Verification items for the finished model (mm, model axes). A direction names the side the tool comes from. Coordinates: 2 decimals unless noted, no trailing zeros. Loops run counter-clockwise (first coordinate to the right, second up) from the corner with the lowest first, then second, coordinate; pieces in that order, holes last. Notation, with made-up numbers: (6, 81) -> (44, 81) arc R17 cw to (44, 101) -> close; hole circle Ø10 at (20.25, -1.75). An arc over 180 degrees is marked (long way). Answer as a JSON object with one key per item and string values. Group by question number.
Q1. Set-up check for faces 1 (the flat face through (-2.938, 0, 37)), 2 (the flat face through (-1, 0, 65)), 3 (the flat face through (2.938, 0, 26)): record each of +Z, -Z, +X, -X, +Y, -Y from which the full face is reachable in a straight line by a thin tool's end or side.
Q2. Gauge pin test, flat ends, axial feed: pin 1 Ø2 at (x, y) = (6, 0.5) entering from +Z; pin 2 Ø2.5 at (x, z) = (-7, 0.83) entering from -Y; pin 3 Ø2.5 at (y, z) = (0, 20.5) entering from +X. Record the tip position at first contact, or that the pin passes through.
Q3. Cross-section at A-A on x = -7. Record the boundary of the cut face in (y, z).
Q4. Cross-section at C-C on y = -1.1. Give the number of separate pieces and of enclosed holes in the cut face, and give its area (3 significant figures).
Q5. Scan lines: L1, parallel to X at y = -0.1, z = 11; L2, parallel to Z at x = -7, y = 2; L3, parallel to Z at x = -0.5, y = 2.1. Record each from-to range of solid material in increasing order.
Q6. Release check for a two-part mould opening along X. For faces 4 (the cylindrical face through (-0.115, -0.035, -0.424)), 5 (the cylindrical face through (4.82, -0.04, 5.92)), 6 (the flat face through (1, -2.5, 26)) record: released by +X, released by -X, zero draft, split by the parting line, or undercut.
Q7. Cross-section at D-D on x = -1.25. Record the boundary of the cut face in (y, z).
Q8. Cross-section at B-B on z = 19. Record the boundary of the cut face in (x, y).
```python
from build123d import *

# Parameters (mm, degrees)
BOSS_EXTRU_1_DEPTH      = 2.5
BOSS_EXTRU_1_DEPTH_BACK = 2.5
ESQUISSE1_R             = 1.5


with BuildPart() as part:
    # Esquisse1 → Boss.-Extru.1 (new, two sides: drawn at the far end of the back side and taken through both)
    with BuildSketch(Plane(origin=(0, 0, 0), x_dir=(1, 0, 0), z_dir=(0, 1, 0)).offset(-BOSS_EXTRU_1_DEPTH_BACK)):
        with BuildLine():
            Line((1.688009203, -65), (-2.938009191, -65))
            Line((-2.938009191, -65), (-2.938009191, -9.008494736))
            ThreePointArc((-2.938009191, -9.008494736), (-4.78031572, -5.95992834), (-7.884337553, -4.212673672))
            ThreePointArc((-7.884337553, -4.212673672), (-10.499981587, -0.814885018), (-7.862349987, 2.565863566))
            ThreePointArc((-7.862349987, 2.565863566), (0, 0.423762079), (7.862349987, 2.565863566))
            ThreePointArc((7.862349987, 2.565863566), (10.499981587, -0.814885018), (7.884337553, -4.212673672))
            ThreePointArc((7.884337553, -4.212673672), (4.78031572, -5.95992834), (2.938009191, -9.008494736))
            Line((2.938009191, -9.008494736), (2.938009191, -43.679635922))
            ThreePointArc((2.938009191, -43.679635922), (2.839937622, -43.977047315), (2.584195047, -44.1577883))
            Line((2.584195047, -44.1577883), (2.041823351, -44.323607971))
            ThreePointArc((2.041823351, -44.323607971), (1.688009203, -44.801760349), (2.041823351, -45.279912727))
            Line((2.041823351, -45.279912727), (2.584195044, -45.445732395))
            ThreePointArc((2.584195044, -45.445732395), (2.839937622, -45.626473379), (2.938009191, -45.923884773))
            ThreePointArc((2.938009191, -45.923884773), (2.839937622, -46.221296165), (2.584195047, -46.40203715))
            Line((2.584195047, -46.40203715), (2.041823351, -46.567856821))
            ThreePointArc((2.041823351, -46.567856821), (1.688009203, -47.046009199), (2.041823351, -47.524161577))
            Line((2.041823351, -47.524161577), (2.584195044, -47.689981245))
            ThreePointArc((2.584195044, -47.689981245), (2.839937622, -47.870722229), (2.938009191, -48.168133623))
            ThreePointArc((2.938009191, -48.168133623), (2.839937622, -48.465545015), (2.584195047, -48.646286))
            Line((2.584195047, -48.646286), (2.041823351, -48.812105672))
            ThreePointArc((2.041823351, -48.812105672), (1.688009203, -49.290258049), (2.041823351, -49.768410427))
            Line((2.041823351, -49.768410427), (2.584195044, -49.934230095))
            ThreePointArc((2.584195044, -49.934230095), (2.839937622, -50.114971079), (2.938009191, -50.412382473))
            ThreePointArc((2.938009191, -50.412382473), (2.839937622, -50.709793865), (2.584195047, -50.89053485))
            Line((2.584195047, -50.89053485), (2.041823351, -51.056354522))
            ThreePointArc((2.041823351, -51.056354522), (1.688009203, -51.5345069), (2.041823351, -52.012659278))
            Line((2.041823351, -52.012659278), (2.584195044, -52.178478945))
            ThreePointArc((2.584195044, -52.178478945), (2.839937622, -52.359219929), (2.938009191, -52.656631323))
            ThreePointArc((2.938009191, -52.656631323), (2.839937622, -52.954042715), (2.584195047, -53.1347837))
            Line((2.584195047, -53.1347837), (2.041823351, -53.300603372))
            ThreePointArc((2.041823351, -53.300603372), (1.688009203, -53.77875575), (2.041823351, -54.256908128))
            Line((2.041823351, -54.256908128), (2.584195044, -54.422727795))
            ThreePointArc((2.584195044, -54.422727795), (2.839937622, -54.603468779), (2.938009191, -54.900880173))
            ThreePointArc((2.938009191, -54.900880173), (2.839937622, -55.198291565), (2.584195047, -55.37903255))
            Line((2.584195047, -55.37903255), (2.041823351, -55.544852222))
            ThreePointArc((2.041823351, -55.544852222), (1.688009203, -56.0230046), (2.041823351, -56.501156978))
            Line((2.041823351, -56.501156978), (2.584195044, -56.666976645))
            ThreePointArc((2.584195044, -56.666976645), (2.839937622, -56.84771763), (2.938009191, -57.145129023))
            ThreePointArc((2.938009191, -57.145129023), (2.839937622, -57.442540415), (2.584195047, -57.6232814))
            Line((2.584195047, -57.6232814), (2.041823351, -57.789101072))
            ThreePointArc((2.041823351, -57.789101072), (1.688009203, -58.26725345), (2.041823351, -58.745405828))
            Line((2.041823351, -58.745405828), (2.584195044, -58.911225495))
            ThreePointArc((2.584195044, -58.911225495), (2.839937622, -59.09196648), (2.938009191, -59.389377873))
            ThreePointArc((2.938009191, -59.389377873), (2.839937622, -59.686789265), (2.584195047, -59.86753025))
            Line((2.584195047, -59.86753025), (2.041823351, -60.033349922))
            ThreePointArc((2.041823351, -60.033349922), (1.688009203, -60.5115023), (2.041823351, -60.989654678))
            Line((2.041823351, -60.989654678), (2.584195044, -61.155474345))
            ThreePointArc((2.584195044, -61.155474345), (2.839937622, -61.33621533), (2.938009191, -61.633626723))
            ThreePointArc((2.938009191, -61.633626723), (2.839937622, -61.931038115), (2.584195047, -62.1117791))
            Line((2.584195047, -62.1117791), (2.041823351, -62.277598772))
            ThreePointArc((2.041823351, -62.277598772), (1.688009203, -62.75575115), (2.041823351, -63.233903528))
            Line((2.041823351, -63.233903528), (2.584195044, -63.399723195))
            ThreePointArc((2.584195044, -63.399723195), (2.839937622, -63.58046418), (2.938009191, -63.877875573))
            ThreePointArc((2.938009191, -63.877875573), (2.839937622, -64.175286965), (2.584195047, -64.35602795))
            Line((2.584195047, -64.35602795), (2.041823351, -64.521847622))
            ThreePointArc((2.041823351, -64.521847622), (1.786080773, -64.702588607), (1.688009203, -65))
        make_face()
        with Locations(Location((7, -0.826237921, 0), (0, 0, 270))):
            Circle(ESQUISSE1_R, mode=Mode.SUBTRACT)
        with Locations(Location((-7, -0.826237921, 0), (0, 0, 90))):
            Circle(ESQUISSE1_R, mode=Mode.SUBTRACT)
    extrude(amount=BOSS_EXTRU_1_DEPTH + BOSS_EXTRU_1_DEPTH_BACK)


solid = part.part
```
Computed values:
{
 "1": {"face 1": "+Z, -X, +Y, -Y", "face 2": "+Z, +X, -X, +Y, -Y", "face 3": "+Z, +X, +Y, -Y"},
 "2": {"pin 1": "stops at z = 5.76", "pin 2": "passes through", "pin 3": "stops at x = 2.94"},
 "3": {"outline": "(-2.5, -2.09) -> (2.5, -2.09) -> (2.5, -0.67) -> (-2.5, -0.67) -> close; (-2.5, 2.33) -> (2.5, 2.33) -> (2.5, 4.51) -> (-2.5, 4.51) -> close"},
 "4": {"separate pieces": "1", "enclosed holes": "2", "area": "455 mm²"},
 "5": {"L1": "x = -2.94 to 2.94", "L2": "z = -2.09 to -0.67, 2.33 to 4.51", "L3": "z = -0.43 to 65"},
 "6": {"face 4": "undercut", "face 5": "released by +X", "face 6": "zero draft"},
 "7": {"outline": "(-2.5, -0.47) -> (2.5, -0.47) -> (2.5, 65) -> (-2.5, 65) -> close"},
 "8": {"outline": "(-2.94, -2.5) -> (2.94, -2.5) -> (2.94, 2.5) -> (-2.94, 2.5) -> close"}
}
